Here's how the part is built. I have some questions about the finished solid (model axes, mm). Give positions to 0.01 mm unless a question says otherwise; leave off trailing zeros. Write each loop counter-clockwise with the first axis right and the second up, starting at its lowest first coordinate (ties: lowest second). Pieces come first, ordered by that corner, then holes. Notation, with made-up numbers: (-39.75, -2) - (-8.75, -2) arc R24 ccw to (-8.75, 22) - close; hole circle Ø3 at (33.5, 64). An arc over 180 degrees is marked (long way). Use one line per item in the form item = value. Start each with the question number.
from build123d import *

# Parameters (mm, degrees)
F2_R      = 5
F0_R      = 2.75
F4_R      = 2.75
F6_FACE_R = 2.75
F8_T      = -0.8


with BuildPart() as f6:
    # F2 (on offset) → F6 section 0
    with BuildSketch(Plane.XY.offset(4)):
        Circle(F2_R)
    # F0 (on Top) → F6 section 1
    with BuildSketch(Plane.XY):
        Circle(F0_R)
    loft()

    # F4 (on offset) → F7 section 0
    with BuildSketch(Plane.XY.offset(-4)):
        Circle(F4_R)
    # F6_face (on face) → F7 section 1
    with BuildSketch(Plane(origin=(0, 0, 0), x_dir=(1, 0, 0), z_dir=(0, 0, -1))):
        Circle(F6_FACE_R)
    loft()

    # F8
    f8_openings = [f6.faces().sort_by_distance(p)[0] for p in [
        (0, 0, 4),
        (0, 0, -4),
    ]]
    offset(amount=F8_T, openings=f8_openings, kind=Kind.INTERSECTION)


solid = f6.part
1. I want a section at A-A, the plane x = 0. List the corners of the cut face in (y, z) for me, then the cut area to 3 significant figures.
2. I want a section at B-B, the plane z = -2.25. List the corners of the cut face in (x, y) for me.
3. We'd pull the mould along Y, two halves only. Please class faces 1 (the face through (-1.437, 1.318, -1.866)), 2 (the face through (1, 2, -4)), 3 (the face through (-0.596, -2.685, -1.972)): pulls with the +Y half, pulls with the -Y half, needs draft (parallel to the pull), parting line crosses it, or undercut.
4. I want a section at C-C, the plane z = 3. List the corners of the cut face in (x, y) for me (1 decimal).
5. Please list where these lines run through material, in increasing order: line 1 (Y direction, x = 0, z = -1.1); line 2 (X direction, y = -3.5, z = 3.75); line 3 (Z direction, x = -2.5, y = -1.5).
6. For P1, Ø4, axis at x = 3, z = -1.5, coming from the -Y side; P2, Ø2, axis at y = 1, z = 3, coming from the +X side; P3, Ø2, axis at x = 3.5, y = 3.5, coming from the -Z side, each with a flat end and sliding along its axis, tell me the tip position at first contact or that it passes through.
Result sheet:
q1.outline = (-5, 4) - (-2.75, 0) - (-2.75, -4) - (-1.95, -4) - (-1.95, 0.21) - (-4.08, 4) - close; (1.95, -4) - (2.75, -4) - (2.75, 0) - (5, 4) - (4.08, 4) - (1.95, 0.21) - close
q1.area = 13.7 mm2
q2.outline = circle Ø5.5 at (0, 0); hole circle Ø3.9 at (0, 0)
q3.face_1 = undercut
q3.face_2 = needs draft
q3.face_3 = parting line crosses it
q4.outline = circle Ø8.9 at (0, 0); hole circle Ø7 at (0, 0)
q5.line_1 = -2.75 to -1.95, 1.95 to 2.75
q5.line_2 = -3.37 to -1.81, 1.81 to 3.37
q5.line_3 = 0.29 to 1.93
q6.P1 = -2.56
q6.P2 = 4.93
q6.P3 = 2.13
